Design review of the part shown in the three views and the two pictorial views. Dimensions are in mm from the part's minimum x, y and z. A direction names the side the tool comes from. Round coordinates to 2 decimals unless told otherwise and drop trailing zeros. Loops run counter-clockwise (first coordinate to the right, second up) from the corner with the lowest first, then second, coordinate; pieces in that order, holes last. Notation, with made-up numbers: (50, -15.75) -> (102, -15.75) arc R6 cw to (102, -9.75) -> close; hole circle Ø10 at (42, 31). An arc over 180 degrees is marked (long way). One line per question, with ' | ' between items. Start each with the question number.
1. For pin 1 Ø1 at (y, z) = (1.5, 1) entering from -X; pin 2 Ø1.5 at (x, y) = (3.5, 1) entering from +Z; pin 3 Ø1.5 at (x, y) = (8, 1) entering from -Z, all flat-tipped, find the tip position at first contact; note any pin that passes through.
2. Consider section B-B (z = 4.5). Write out the cut boundary in (x, y), and give its area (3 significant figures).
3. For the marked faces 1 and 2, list the 3-axis set-ups (+Z, -Z, +X, -X, +Y, -Y) from which the entire face can be reached by the end or side of a thin tool; tool diameter is ignored.
4. Consider section C-C (y = 1). Write out the cut boundary in (x, z).
5. Wall thickness on line 1 along Z through (x, y) = (4.5, 1.25); line 2 along X through (y, z) = (1.2, 3.25); line 3 along Y through (x, z) = (7.25, 2.75): over which ranges is each line inside the solid? List them lowest first.
6. Draft analysis for pull direction Z (two halves, no side actions). For the marked faces 3, 4 and 5, state which applies: pulls with the +Z half, pulls with the -Z half, needs draft (parallel to the pull), parting line crosses it, or undercut.
7. Consider section A-A (x = 4.5). Write out the cut boundary in (y, z).
8. Consider section D-D (y = 1.85). Write out the cut boundary in (x, z), and give its area (3 significant figures).
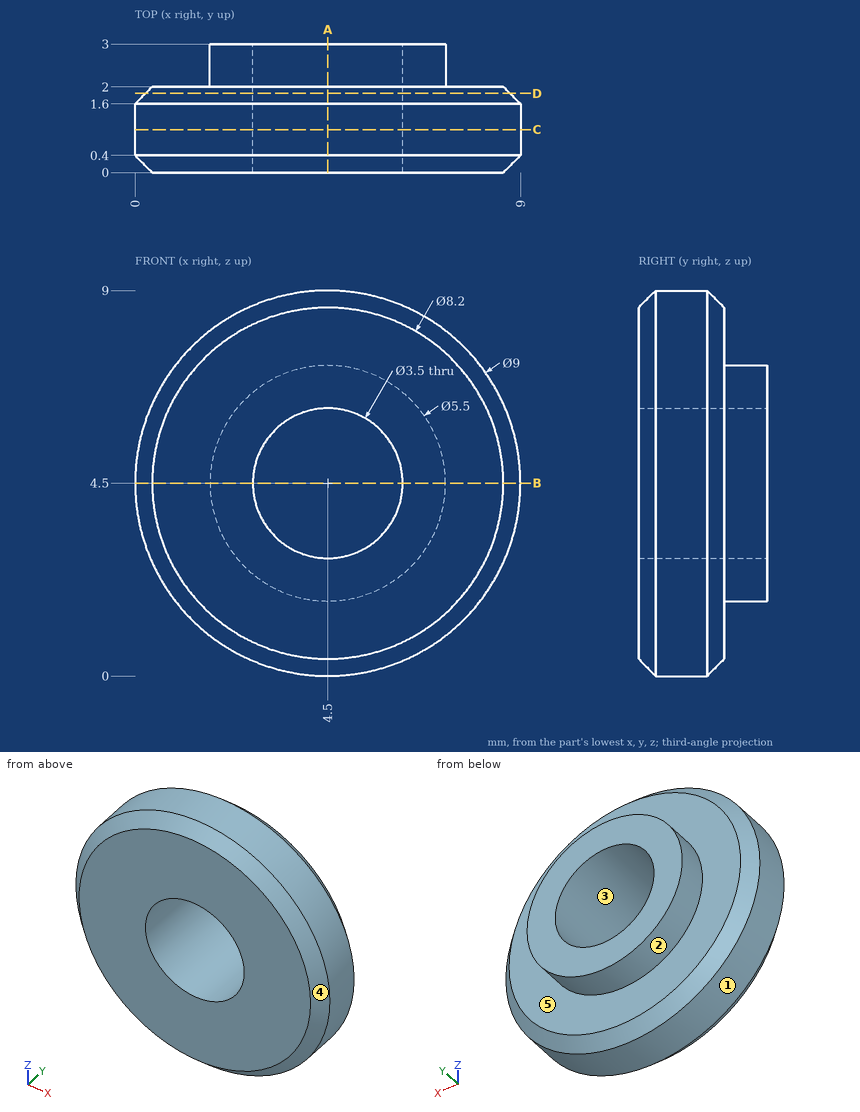
Answer block:
1) pin 1: stops at x = 1.15 | pin 2: stops at z = 8.99 | pin 3: stops at z = 0.94
2) outline: (0, 0.4) -> (0.4, 0) -> (2.75, 0) -> (2.75, 3) -> (1.75, 3) -> (1.75, 2) -> (0.4, 2) -> (0, 1.6) -> close; (6.25, 0) -> (8.6, 0) -> (9, 0.4) -> (9, 1.6) -> (8.6, 2) -> (7.25, 2) -> (7.25, 3) -> (6.25, 3) -> close | area: 12.7 mm2
3) face 1: +Y, -Y | face 2: +Y
4) outline: circle Ø9 at (4.5, 4.5); hole circle Ø3.5 at (4.5, 4.5)
5) line 1: z = 0 to 2.75, 6.25 to 9 | line 2: x = 0.18 to 3.28, 5.72 to 8.82 | line 3: y = 0 to 2
6) face 3: undercut | face 4: parting line crosses it | face 5: needs draft
7) outline: (0, 0.4) -> (0.4, 0) -> (1.6, 0) -> (2, 0.4) -> (2, 1.75) -> (3, 1.75) -> (3, 2.75) -> (0, 2.75) -> close; (0, 6.25) -> (3, 6.25) -> (3, 7.25) -> (2, 7.25) -> (2, 8.6) -> (1.6, 9) -> (0.4, 9) -> (0, 8.6) -> close
8) outline: circle Ø8.5 at (4.5, 4.5); hole circle Ø3.5 at (4.5, 4.5) | area: 47.1 mm2
